Verification items for this drawing (mm, ordinates from the low corner). A direction names the side the tool comes from. Round coordinates to 2 decimals unless told otherwise and drop trailing zeros. Order: outer loops, then holes, each group sorted by start corner. A loop starts at its lowest first (then second) coordinate and runs counter-clockwise, first axis right, second up. Notation, with made-up numbers: (7.5, 73) -> (37.5, 73) arc R20 ccw to (37.5, 112) -> close; hole circle Ø2 at (-31.5, -31.5). An arc over 180 degrees is marked (long way). Answer in a Markdown table with one row per item. Add a question column.
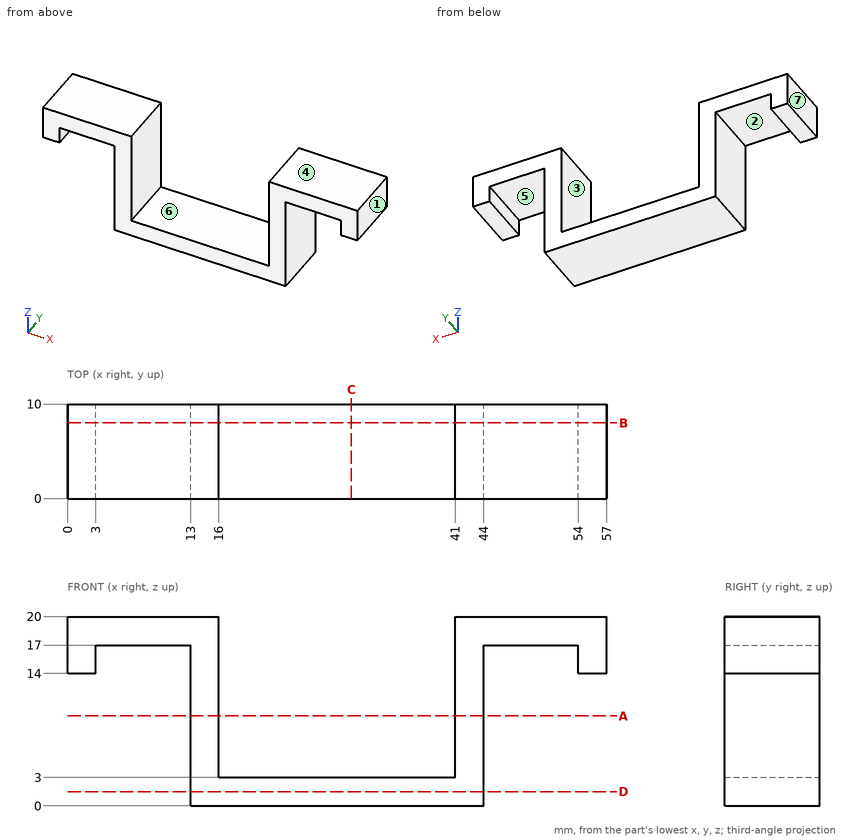
1) Cross-section at D-D, the plane z = 1.5. Record the boundary of the cut face in (x, y), and give its area (3 significant figures).
2) Draft check along X on the marked faces 4, 5, 6 and 7. Enter one of: +X half, -X half, draft (parallel to the pull), parting line (faces both ways), or undercut.
3) Cross-section at B-B, the plane y = 8. Record the boundary of the cut face in (x, z), and give its area (3 significant figures).
4) Thickness scan on L1, parallel to X at y = 2, z = 15.75; L2, parallel to X at y = 1.5, z = 11.5; L3, parallel to X at y = 2.5, z = 17.25. Record the ranges inside material, lowest first. Write a range as [from, to].
5) Cross-section at C-C, the plane x = 30. Record the boundary of the cut face in (y, z).
6) Depth check by flat-ended pin: P1, Ø3, axis at y = 6.5, z = 7.5, coming from the -X side; P2, Ø5, axis at x = 51, y = 3.5, coming from the -Z side; P3, Ø0.9, axis at x = 1, y = 5, coming from the -Z side. Enter the tip coordinate at first touch or a pass-through.
7) Cross-section at A-A, the plane z = 9.5. Record the boundary of the cut face in (x, y), and give its area (3 significant figures).
8) Tool access check on the marked faces 1, 2 and 3. Record the directions out of +Z, -Z, +X, -X, +Y, -Y that give a thin tool (end or side, any length) a straight path to the whole face; none if there is none.
Results below:
| question | item | result |
|---|---|---|
| 1 | outline | (13, 0) -> (44, 0) -> (44, 10) -> (13, 10) -> close |
| 1 | area | 310 mm² |
| 2 | face 4 | draft |
| 2 | face 5 | undercut |
| 2 | face 6 | undercut |
| 2 | face 7 | -X half |
| 3 | outline | (0, 14) -> (3, 14) -> (3, 17) -> (13, 17) -> (13, 0) -> (44, 0) -> (44, 17) -> (54, 17) -> (54, 14) -> (57, 14) -> (57, 20) -> (41, 20) -> (41, 3) -> (16, 3) -> (16, 20) -> (0, 20) -> close |
| 3 | area | 291 mm² |
| 4 | L1 | [0, 3], [13, 16], [41, 44], [54, 57] |
| 4 | L2 | [13, 16], [41, 44] |
| 4 | L3 | [0, 16], [41, 57] |
| 5 | outline | (0, 0) -> (10, 0) -> (10, 3) -> (0, 3) -> close |
| 6 | P1 | x = 13 |
| 6 | P2 | z = 17 |
| 6 | P3 | z = 14 |
| 7 | outline | (13, 0) -> (16, 0) -> (16, 10) -> (13, 10) -> close; (41, 0) -> (44, 0) -> (44, 10) -> (41, 10) -> close |
| 7 | area | 60.0 mm² |
| 8 | face 1 | +Z, -Z, +X, +Y, -Y |
| 8 | face 2 | -Z, +Y, -Y |
| 8 | face 3 | +Z, +Y, -Y |
